from build123d import *

# Parameters (mm, degrees)
F0_R          = 11
F0_R_2        = 4.15
F1_DEPTH      = 25
F2_R          = 9.5
F2_R_2        = 4.15
F3_DEPTH      = 70
F4_R          = 4.15
F5_DEPTH      = 11.001
F5_DEPTH_BACK = 25
F6_R          = 4.15
F7_DEPTH      = 37
F8_R          = 8
F9_DEPTH      = 39
F10_R         = 1.5
F11_W         = 4.6595567837
F11_H         = 11.4234238863
F12_DEPTH     = 25


with BuildPart() as f1:
    # F0 (on Front) → F1 (new body)
    with BuildSketch(Plane.XZ):
        Circle(F0_R)
        Circle(F0_R_2, mode=Mode.SUBTRACT)
    extrude(amount=F1_DEPTH)

    # F2 (on face) → F3 (join)
    with BuildSketch(Plane(origin=(0, 0, 0), x_dir=(-1, 0, 0), z_dir=(0, 1, 0))):
        Circle(F2_R)
        Circle(F2_R_2, mode=Mode.SUBTRACT)
        Circle(F2_R_2)
    extrude(amount=F3_DEPTH)

    # F4 (on Top) → F5 (cut, two sides)
    with BuildSketch(Plane.XY) as f5_sk:
        with Locations((0, 12)):
            Circle(F4_R)
    extrude(amount=F5_DEPTH, mode=Mode.SUBTRACT)
    extrude(f5_sk.sketch, amount=-F5_DEPTH_BACK, mode=Mode.SUBTRACT)

    # F6 (on face) → F7 (cut)
    with BuildSketch(Plane.XZ.offset(25)):
        Circle(F6_R)
    extrude(amount=-F7_DEPTH, mode=Mode.SUBTRACT)

    # F8 (on face) → F9 (join)
    with BuildSketch(Plane(origin=(0, 70, 0), x_dir=(-1, 0, 0), z_dir=(0, 1, 0))):
        Circle(F8_R)
    extrude(amount=F9_DEPTH)

    # F10
    f10_edges = [f1.edges().sort_by_distance(p)[0] for p in [
        (8, 109, 0),
    ]]
    fillet(f10_edges, radius=F10_R)

    # F11 (on Top) → F12 (cut)
    with BuildSketch(Plane.XY):
        with Locations((-2.3297783919, 90.184956789)):
            Rectangle(F11_W, F11_H)
    extrude(amount=F12_DEPTH, mode=Mode.SUBTRACT)


solid = f1.part
Geometry check sheet. Reference: the model listing, model coordinates, mm. A direction names the side the tool comes from. Coordinates: 2 decimals unless noted, no trailing zeros. Order: outer loops, then holes, each group sorted by start corner. A loop starts at its lowest first (then second) coordinate and runs counter-clockwise, first axis right, second up. Notation, with made-up numbers: (-38, 81.5) -> (-18, 81.5) arc R13 cw to (-18, 100.5) -> close; hole circle Ø2 at (-7.75, 84.25). An arc over 180 degrees is marked (long way). Use a Markdown table: item, result. Add a question column.
1. Material ranges on L1, parallel to Z at x = 0, y = 3.75; L2, parallel to Z at x = 0, y = -6.5; L3, parallel to Y at x = 0.25, z = 8.75, recorded low to high.
2. Go/stop test with flat-tipped pins: pin 1 Ø1.4 at (x, y) = (-3.5, 91.5) entering from +Z; pin 2 Ø5 at (y, z) = (87.5, 3.5) entering from +X; pin 3 Ø2 at (y, z) = (88.5, 4.5) entering from -X. Record where each tip stops, or that it passes through.
3. Cross-section at A-A (y = -11). Enter the section's corners in (x, z), and give its area (3 significant figures).
4. Cross-section at C-C (y = 66). Enter the section's corners in (x, z), and give its area (3 significant figures).
5. Cross-section at B-B (x = 3). Give the number of separate pieces and of enclosed holes in the cut face, and give its area (3 significant figures).
6. Mould release check, pull along X, two halves, no side actions. Record for faces 1 (the face through (0, -25, -5)), 2 (the face through (1.73, 88.49, -7.81)), 3 (the face through (-4.66, 90, 3)): pulls with the +X half, pulls with the -X half, needs draft (parallel to the pull), parting line crosses it, or undercut.
7. Set-up check for faces 4 (the face through (-2.38, -12.32, -10.74)), 5 (the face through (4.3, 70, -7)), 6 (the face through (0, 90, 4)): record each of +Z, -Z, +X, -X, +Y, -Y from which the full face is reachable in a straight line by a thin tool's end or side.
Filled sheet:
| question | item | result |
|---|---|---|
| 1 | L1 | -9.5 to -4.15, 4.15 to 9.5 |
| 1 | L2 | -11 to -4.15, 4.15 to 11 |
| 1 | L3 | -25 to 7.86, 16.14 to 70 |
| 2 | pin 1 | z = 0 |
| 2 | pin 2 | x = 7.94 |
| 2 | pin 3 | x = -7.19 |
| 3 | outline | circle Ø22 at (0, 0); hole circle Ø8.3 at (0, 0) |
| 3 | area | 326 mm2 |
| 4 | outline | circle Ø19 at (0, 0) |
| 4 | area | 284 mm2 |
| 5 | separate pieces | 3 |
| 5 | enclosed holes | 0 |
| 5 | area | 2,070 mm2 |
| 6 | face 1 | needs draft |
| 6 | face 2 | parting line crosses it |
| 6 | face 3 | undercut |
| 7 | face 4 | +Y, -Y |
| 7 | face 5 | +Y |
| 7 | face 6 | +Z |
